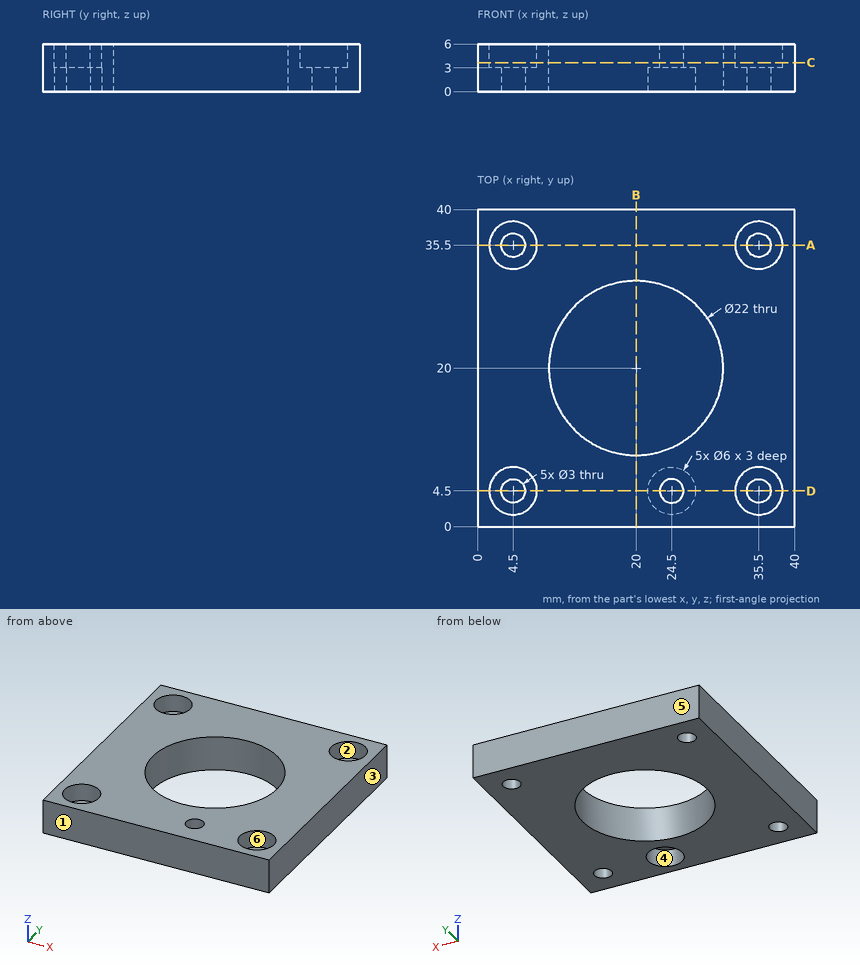
Job drawing, mm, ordinate dimensions from the low corner. One solid piece. A direction names the side the tool comes from. Coordinates: 2 decimals unless noted, no trailing zeros. Write each loop counter-clockwise with the first axis right and the second up, starting at its lowest first coordinate (ties: lowest second). Pieces come first, ordered by that corner, then holes. Notation, with made-up numbers: M 32,-34.75 L 43,-34.75 A24 cw 43,3.25 Z; hole C 47,-21.75 d4. An arc over 180 degrees is marked long. Answer as a JSON object with one key per item and string values. Group by question number.
1) Pin check, flat tips, straight feed: pin 1 Ø3.5 at (x, y) = (35.5, 4.5) entering from -Z; pin 2 Ø5 at (x, y) = (4.5, 4.5) entering from +Z; pin 3 Ø3.5 at (x, y) = (24.5, 4.5) entering from -Z. Stop position of each tip, or through.
2) Tool access for the marked faces 5 and 6: list every direction of +Z, -Z, +X, -X, +Y, -Y with a clear straight run to the whole face (end or side of a thin tool).
3) Saw through at A-A (y = 35.5). Write the cut outline in (x, z), plus the area to 3 significant figures.
4) Saw through at C-C (z = 3.65). Write the cut outline in (x, y), plus the area to 3 significant figures.
5) Mould opens along X. For the marked faces 1, 2, 3 and 4 say: +X half, -X half, draft (parallel to the pull), parting line (faces both ways), or undercut.
6) Wall check: line 1 (Y direction, x = 35.5, z = 5.05); line 2 (Y direction, x = 5.5, z = 3.5); line 3 (Y direction, x = 20, z = 5.5). Give the ranges that are in metal, low to high. Write a range as from..to.
7) Saw through at D-D (y = 4.5). Write the cut outline in (x, z), plus the area to 3 significant figures.
8) Saw through at B-B (x = 20). Write the cut outline in (y, z).
Values follow:
{
 "1": {"pin 1": "stops at z = 0", "pin 2": "stops at z = 3", "pin 3": "stops at z = 3"},
 "2": {"face 5": "+Z, -Z, +X, -X, +Y", "face 6": "+Z"},
 "3": {"outline": "M 0,0 L 3,0 L 3,3 L 1.5,3 L 1.5,6 L 0,6 Z; M 6,0 L 34,0 L 34,3 L 32.5,3 L 32.5,6 L 7.5,6 L 7.5,3 L 6,3 Z; M 37,0 L 40,0 L 40,6 L 38.5,6 L 38.5,3 L 37,3 Z", "area": "186 mm2"},
 "4": {"outline": "M 0,0 L 40,0 L 40,40 L 0,40 Z; hole C 4.5,4.5 d6; hole C 4.5,35.5 d6; hole C 20,20 d22; hole C 24.5,4.5 d3; hole C 35.5,4.5 d6; hole C 35.5,35.5 d6", "area": "1,100 mm2"},
 "5": {"face 1": "draft", "face 2": "undercut", "face 3": "+X half", "face 4": "undercut"},
 "6": {"line 1": "y = 0..1.5, 7.5..32.5, 38.5..40", "line 2": "y = 0..1.67, 7.33..32.67, 38.33..40", "line 3": "y = 0..9, 31..40"},
 "7": {"outline": "M 0,0 L 3,0 L 3,3 L 1.5,3 L 1.5,6 L 0,6 Z; M 6,0 L 21.5,0 L 21.5,3 L 23,3 L 23,6 L 7.5,6 L 7.5,3 L 6,3 Z; M 26,3 L 27.5,3 L 27.5,0 L 34,0 L 34,3 L 32.5,3 L 32.5,6 L 26,6 Z; M 37,0 L 40,0 L 40,6 L 38.5,6 L 38.5,3 L 37,3 Z", "area": "159 mm2"},
 "8": {"outline": "M 0,0 L 9,0 L 9,6 L 0,6 Z; M 31,0 L 40,0 L 40,6 L 31,6 Z"}
}
